For this review, take the finished solid that the model builds, in its own axes (mm). Face numbers are marked on the shaded views. A direction names the side the tool comes from. Coordinates: 2 decimals unless noted, no trailing zeros. Loops run counter-clockwise (first coordinate to the right, second up) from the corner with the lowest first, then second, coordinate; pieces in that order, holes last. Notation, with made-up numbers: M -37,38 L -1,38 A31 cw -1,75 Z; hole C 14.5,23.25 d4. An arc over 180 degrees is marked long. Write item = value, one per line.
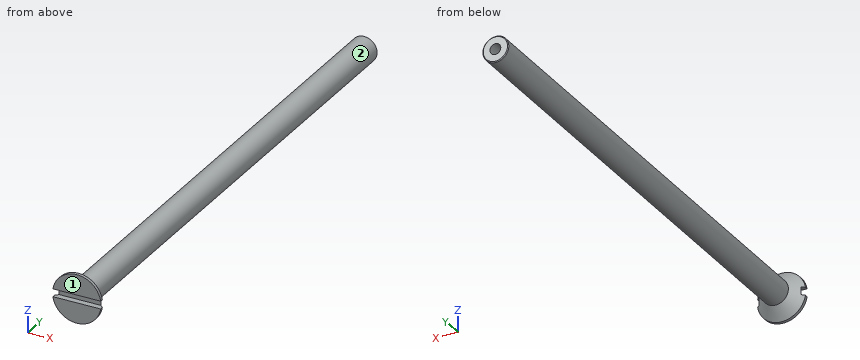
from build123d import *

# Parameters (mm, degrees)
SKETCH_1_R               = 1.5
EXTRUDE_1_DEPTH          = 61
SKETCH_3_W               = 0.9
SKETCH_3_H               = 0.7
CUT_EXTRUDE_1_DEPTH      = 3.8
CUT_EXTRUDE_1_DEPTH_BACK = 3.8
CHAMFER_1_SIZE           = 0.1
HOLE_WIZARD_M1_61_D      = 1.25
HOLE_WIZARD_M1_61_DEPTH  = 7
HOLE_WIZARD_M1_61_TIP    = 0.375537887


with BuildPart() as part:
    # Эскиз1 → Бобышка-Вытянуть1 (new body)
    with BuildSketch(Plane(origin=(0, 0, 0), x_dir=(1, 0, 0), z_dir=(0, 1, 0))):
        Circle(SKETCH_1_R)
    extrude(amount=EXTRUDE_1_DEPTH)

    # Эскиз2 → Повернуть1 (revolve)
    with BuildSketch(Plane(origin=(0, 0, 0), x_dir=(0, 0, -1), z_dir=(1, 0, 0))):
        Polygon((0, 3.15), (-2.8, 0.35), (-2.8, 0), (0, 0), align=None)
    revolve(axis=Axis((0, 0, 0), (0, 1, 0)))

    # Эскиз3 → Вырез-Вытянуть1 (cut, two sides)
    with BuildSketch(Plane(origin=(0, 0, 0), x_dir=(0, 0, -1), z_dir=(1, 0, 0))) as cut_extrude_1_sk:
        with Locations((0, 0.35)):
            Rectangle(SKETCH_3_W, SKETCH_3_H)
    extrude(amount=CUT_EXTRUDE_1_DEPTH, mode=Mode.SUBTRACT)
    extrude(cut_extrude_1_sk.sketch, amount=-CUT_EXTRUDE_1_DEPTH_BACK, mode=Mode.SUBTRACT)

    # Фаска1
    chamfer_1_edges = [part.edges().sort_by_distance(p)[0] for p in [
        (-1.5, 61, 0),
    ]]
    chamfer(chamfer_1_edges, length=CHAMFER_1_SIZE)

    # Отверстие обработанное метчиком M1,61
    with Locations(Plane(origin=(0, 61, 0), x_dir=(1, 0, 0), z_dir=(0, 1, 0))):
        with Locations((0, 0)):
            Hole(HOLE_WIZARD_M1_61_D / 2, depth=HOLE_WIZARD_M1_61_DEPTH)
            with Locations((0, 0, -(HOLE_WIZARD_M1_61_DEPTH + HOLE_WIZARD_M1_61_TIP / 2))):  # 118° drill point
                Cone(0, HOLE_WIZARD_M1_61_D / 2, HOLE_WIZARD_M1_61_TIP, mode=Mode.SUBTRACT)


solid = part.part
Q1. Machinability: for the marked faces 1 and 2, which of the approach directions +Z, -Z, +X, -X, +Y, -Y give a long, thin tool a straight path to every point of the face, cutting with its end or side? Answer none if there is none.
Solved:
face_1 = +Z, -Z, +X, -X, -Y
face_2 = +Y
Q2. For pin 1 Ø3 at (x, y) = (1, 31.5) entering from -Z; pin 2 Ø0.6 at (x, y) = (-0.5, 0) entering from +Z; pin 3 Ø0.8 at (x, z) = (0, 0) entering from -Y, all flat-tipped, find the tip position at first contact; note any pin that passes through.
Solved:
pin_1 = -1.5
pin_2 = 2.79
pin_3 = 0.7
Q3. Add section A-A (y = 55). Write out the cut boundary in (x, z) (3 decimals), and give its area (3 significant figures).
Solved:
outline = C 0,0 d3; hole C 0,0 d1.25
area = 5.84 mm²
Q4. For line 1 along Z through (x, y) = (0, 56.75) (3 decimals); line 2 along Y through (x, z) = (-0.5, -2.4); line 3 along Y through (x, z) = (-1.1, 0.25), list the stretches that pass through material, from the lowest coordinate up.
Solved:
line_1 = -1.5 to -0.625, 0.625 to 1.5
line_2 = 0 to 0.7
line_3 = 0.7 to 61
Q5. Add section B-B (y = 17.5). Write out the cut boundary in (x, z).
Solved:
outline = C 0,0 d3
